Autodesk Fusion 360 part; units mm, degrees
sketch "Sketch1" plane through (0, 0, 0) normal (1, 0, 0) x (0, 1, 0)
  line L0 (0, 0) -> (50, 0) construction
  line L1 (0, 0) -> (0, 21) construction
  line L2 (0, 21) -> (20, 21) construction
  line L3 (0, 0) -> (20, 21) construction
  line L4 (20, 21) -> (50, 0) construction
  line L5 (50, 0) -> (80, 0) construction
  line L6 (20, 21) -> (80, 21) construction
  line L7 (50, 0) -> (80, 21) construction
  line L8 (80, 0) -> (80, 21) construction
  line L9 (7.8851, 5.3793) -> (19.0759, 17.1297)
  line L10 (62.6895, 2) -> (80, 2)
  line L11 (9.3333, 2) -> (37.3105, 2)
  line L12 (31.5425, 15.3615) -> (48.8531, 3.2442)
  line L13 (21.6711, 17.3889) -> (38.4575, 5.6385)
  line L14 (61.5425, 5.6385) -> (80, 18.5587)
  line L15 (0, -2) -> (50, -2)
  line L16 (50, -2) -> (80, -2)
  line L17 (20, 23) -> (80, 23)
  line L18 (-1.4483, 1.3793) -> (18.5517, 22.3793)
  line L19 (32.6895, 19) -> (67.3105, 19)
  line L20 (51.1469, 3.2442) -> (68.4575, 15.3615)
  arc A0 (20, 23) -> (18.5517, 22.3793) centre (20, 21) ccw
  arc A1 (-1.4483, 1.3793) -> (0, -2) centre (0, 0) ccw
  arc A2 (21.6711, 17.3889) -> (19.0759, 17.1297) centre (20.5242, 15.7504) ccw
  arc A3 (7.8851, 5.3793) -> (9.3333, 2) centre (9.3333, 4) ccw
  arc A4 (37.3105, 2) -> (38.4575, 5.6385) centre (37.3105, 4) ccw
  arc A5 (32.6895, 19) -> (31.5425, 15.3615) centre (32.6895, 17) ccw
  arc A6 (68.4575, 15.3615) -> (67.3105, 19) centre (67.3105, 17) ccw
  arc A7 (48.8531, 3.2442) -> (51.1469, 3.2442) centre (50, 4.8826) ccw
  arc A8 (61.5425, 5.6385) -> (62.6895, 2) centre (62.6895, 4) ccw
  line L21 (80, 18.5587) -> (80, 23)
  line L22 (80, 2) -> (80, -2)
  dimension "d52" = 50
  dimension "d53" = 21
  dimension "d54" = 20
  dimension "d55" = 30
  dimension "d56" = 60
  dimension "d61" = 25
  dimension "d62" = 4
  dimension "d63" = 2
  dimension "d64" = 2
  dimension "d65" = 4
  dimension "d66" = 4
  dimension "d67" = 2
  dimension "d68" = 4
  dimension "d69" = 2
  dimension "d70" = 4
  dimension "d71" = 2
  dimension "d73" = 4
  dimension "d74" = 2
  dimension "d75" = 2
  dimension "d76" = 2
  dimension "d77" = 2
  dimension "d78" = 2
  dimension "d79" = 2
  dimension "d80" = 2
  dimension "d81" = 2
  dimension "d82" = 2
extrude "Extrude2" add sketch "Sketch1" along normal blind 14 makes body 1
ref_plane "WorkPlane1" through (0, 80, 0) normal (0, 1, 0) x (0, 0, 1)
mirror "Mirror1" about plane through (0, 80, 0) normal (0, 1, 0) of bodies 1 merged
copy_body "Body->Comp3" bodies 1 removing the originals makes body 2 in component "Truss Half"
component "Truss Half" placed x (1, 0, 0) y (0, 1, 0) z (0, 0, 1) at (0, 0, 0)
Geometry: final body of the model. Coordinates: model frame, mm. A direction names the side the tool comes from. Round coordinates to 2 decimals unless told otherwise and drop trailing zeros. Loops run counter-clockwise (first coordinate to the right, second up) from the corner with the lowest first, then second, coordinate; pieces in that order, holes last. Notation, with made-up numbers: M 41,-15.75 L 97,-15.75 A24 ccw 97,0.25 Z; hole C 2.25,46 d2. An arc over 180 degrees is marked long. Put each result on its own line as item: value. Start each with the question number.
(1) Set-up query: faces 4 (the face through (7, 79, 23)), 5 (the face through (6.902, 59.681, 9.218)). Return all of +Z, -Z, +X, -X, +Y, -Y with unobstructed straight access to the full face (end or side cutting, diameter ignored); none if empty.
(2) Section query D-D (x = 9.75). State how many separate pieces and enclosed holes the cut face has, then the cut area to 3 significant figures.
(3) Contact query for flat-ended pins moving along their axis: pin 1 Ø6 at (x, z) = (9.5, 9.5) entering from -Y; pin 2 Ø10 at (y, z) = (69.5, 7) entering from +X; pin 3 Ø1 at (x, z) = (3.5, 11.5) entering from +Y. Output: stop coordinate, or through.
(4) Section query B-B (y = 74). Return loops of the section in (x, z).
(5) Section query A-A (z = 7.75). Return loops of the section in (x, y), then the cut area to 3 significant figures.
(6) Material intervals for line 1 along Y through (x, z) = (9.25, 12.75); line 2 along Z through (x, y) = (8.75, 97); line 3 along Y through (x, z) = (8.25, 16.5), sorted ascending. Write a range as [from, to].
(7) Section query C-C (y = 124.5). Return loops of the section in (x, z).
(8) Draft query along Y for faces 1 (the face through (6.9, 69.21, 17.63)), 2 (the face through (7, 79, -2)), 3 (the face through (6.902, 151.308, 12.026)). Return one class per face: +Y half, -Y half, draft (parallel to the pull), parting line (faces both ways), or undercut.
Findings below:
1. face 4: +Z, +X, -X, +Y, -Y
1. face 5: +X, -X
2. separate pieces: 1
2. enclosed holes: 5
2. area: 1,890 mm2
3. pin 1: stops at y = 3.43
3. pin 2: stops at x = 14
3. pin 3: stops at y = 152.29
4. outline: M 0,-2 L 14,-2 L 14,2 L 0,2 Z; M 0,14.36 L 14,14.36 L 14,23 L 0,23 Z
5. outline: M 0,4.62 L 14,4.62 L 14,10.14 L 0,10.14 Z; M 0,35.44 L 14,35.44 L 14,42.42 L 0,42.42 Z; M 0,57.58 L 14,57.58 L 14,64.56 L 0,64.56 Z; M 0,95.44 L 14,95.44 L 14,102.42 L 0,102.42 Z; M 0,117.58 L 14,117.58 L 14,124.56 L 0,124.56 Z; M 0,149.86 L 14,149.86 L 14,155.38 L 0,155.38 Z
5. area: 545 mm2
6. line 1: y = [9.38, 14.9], [28.3, 35.27], [64.73, 71.7], [88.3, 95.27], [124.73, 131.7], [145.1, 150.62]
6. line 2: z = [-2, 2], [6.66, 11.54], [19, 23]
6. line 3: y = [12.95, 18.48], [22.94, 30.75], [69.25, 77.06], [82.94, 90.75], [129.25, 137.06], [141.52, 147.05]
7. outline: M 0,-2 L 14,-2 L 14,2 L 0,2 Z; M 0,7.71 L 14,7.71 L 14,12.59 L 0,12.59 Z; M 0,19 L 14,19 L 14,23 L 0,23 Z
8. face 1: undercut
8. face 2: draft
8. face 3: +Y half
